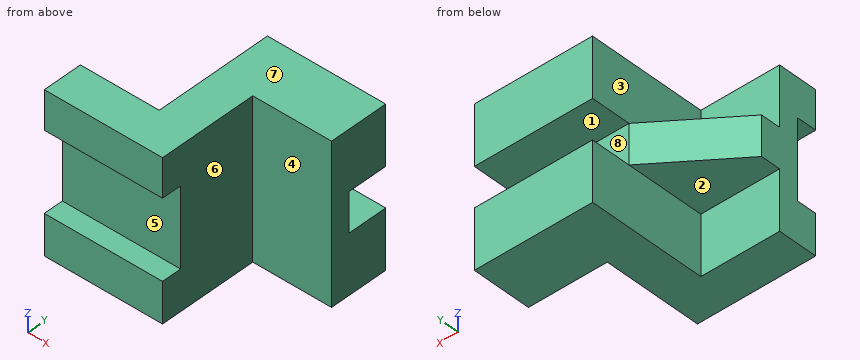
from build123d import *

# Parameters (mm, degrees)
BOSS_EXTRUDE1_DEPTH = 40
CUT_EXTRUDE1_DEPTH  = 30
CUT_EXTRUDE2_DEPTH  = 30
CUT_EXTRUDE3_REACH  = 62
SKETCH4_W           = 20
SKETCH4_H           = 20.212765958
CUT_EXTRUDE4_REACH  = 102
SKETCH5_W           = 40
SKETCH5_H           = 10


with BuildPart() as part:
    # Sketch1 → Boss-Extrude1 (new body, symmetric)
    with BuildSketch(Plane.XY):
        Polygon((-14.731740416, -28.723404255), (-14.731740416, 11.063829787), (-14.731740416, 31.276595745), (45.268259584, 31.276595745), (45.268259584, 1.276595745), (5.268259584, 1.276595745), (5.268259584, -48.723404255), (-54.731740416, -48.723404255), (-54.731740416, -28.723404255), align=None)
        Polygon((-54.731740416, -28.723404255), (-14.731740416, -28.723404255), (-14.731740416, 11.063829787), (-54.731740416, -18.723404255), align=None)
    extrude(amount=BOSS_EXTRUDE1_DEPTH, both=True)

    # Sketch2 → Cut-Extrude1 (cut)
    with BuildSketch(Plane.XY.offset(40)):
        Polygon((-54.731740416, -18.723404255), (-54.731740416, -28.723404255), (-14.731740416, -28.723404255), (-14.731740416, 11.063829787), align=None)
    extrude(amount=-CUT_EXTRUDE1_DEPTH, mode=Mode.SUBTRACT)

    # Sketch3 → Cut-Extrude2 (cut)
    with BuildSketch(Plane(origin=(0, 0, -40), x_dir=(-1, 0, 0), z_dir=(0, 0, -1))):
        Polygon((14.731740416, 11.063829787), (54.731740416, -18.723404255), (54.731740416, -28.723404255), (14.731740416, -28.723404255), align=None)
    extrude(amount=-CUT_EXTRUDE2_DEPTH, mode=Mode.SUBTRACT)

    # Sketch4 → Cut-Extrude3 (cut, up to next)
    with BuildSketch(Plane.ZY.offset(14.731740416), mode=Mode.PRIVATE) as cut_extrude3_sk1:
        with Locations((0, 21.170212766)):
            Rectangle(SKETCH4_W, SKETCH4_H)
    cut_extrude3_tool1 = extrude(cut_extrude3_sk1.sketch, amount=-CUT_EXTRUDE3_REACH, mode=Mode.PRIVATE) & part.part
    add(cut_extrude3_tool1.solids().sort_by_distance((-14.73174, 21.170213, 0))[0], mode=Mode.SUBTRACT)

    # Sketch5 → Cut-Extrude4 (cut, up to next)
    with BuildSketch(Plane.ZY.offset(54.731740416), mode=Mode.PRIVATE) as cut_extrude4_sk1:
        with Locations((0.497624841, -43.723404255)):
            Rectangle(SKETCH5_W, SKETCH5_H)
    cut_extrude4_tool1 = extrude(cut_extrude4_sk1.sketch, amount=-CUT_EXTRUDE4_REACH, mode=Mode.PRIVATE) & part.part
    add(cut_extrude4_tool1.solids().sort_by_distance((-54.73174, -43.723404, 0.497625))[0], mode=Mode.SUBTRACT)


solid = part.part
Geometry: final body of the model. Coordinates: model frame, mm. Face numbers are marked on the shaded views. A direction names the side the tool comes from. Coordinates: 2 decimals unless noted, no trailing zeros. Order: outer loops, then holes, each group sorted by start corner. A loop starts at its lowest first (then second) coordinate and runs counter-clockwise, first axis right, second up.
1) First-contact query: P1, Ø20, axis at x = 34, z = -17.5, coming from the -Y side; P2, Ø3, axis at y = -7, z = -11, coming from the +X side; P3, Ø12, axis at x = 10.5, z = 31.5, coming from the -Y side; P4, Ø20, axis at x = -26.5, y = -10.5, coming from the +Z side. Flat tips, straight axial feed; report the tip coordinate or a pass-through.
Result sheet:
P1: stops at y = 1.28
P2: stops at x = 5.27
P3: stops at y = -48.72
P4: stops at z = 10
2) Section A-A (y = 22.5). Return loops of the section in (x, z), then the cut area to 3 significant figures.
Result sheet:
outline: (-14.73, -40) - (45.27, -40) - (45.27, -10) - (-14.73, -10) - close; (-14.73, 10) - (45.27, 10) - (45.27, 40) - (-14.73, 40) - close
area: 3,600 mm2
3) Set-up query: the marked faces 1, 2, 3 and 4. Return all of +Z, -Z, +X, -X, +Y, -Y with unobstructed straight access to the full face (end or side cutting, diameter ignored); none if empty.
Result sheet:
face 1: +X, -X, +Y
face 2: -Z, -X, +Y
face 3: +Z, -X, +Y
face 4: +Z, -Z, +X, -Y
4) Section C-C (y = -22.5). Return loops of the section in (x, z), then the cut area to 3 significant figures.
Result sheet:
outline: (-54.73, -10) - (-14.73, -10) - (-14.73, -40) - (5.27, -40) - (5.27, 40) - (-14.73, 40) - (-14.73, 10) - (-54.73, 10) - close
area: 2,400 mm2
5) Draft query along Z for the marked faces 5, 6, 7 and 8. Return one class per face: released by +Z, released by -Z, zero draft, split by the parting line, or undercut.
Result sheet:
face 5: undercut
face 6: zero draft
face 7: released by +Z
face 8: undercut
6) Ray query, probe 1 along Z at (x, y) = (34, 17); probe 2 along Z at (x, y) = (-37, -45); probe 3 along Y at (x, z) = (-50, 30.5). Return the intervals inside material, ascending.
Result sheet:
probe 1: z = -40 to -10, 10 to 40
probe 2: z = -40 to -19.5, 20.5 to 40
probe 3: y = -48.72 to -28.72
7) Section B-B (z = -5.5). Return loops of the section in (x, y), then the cut area to 3 significant figures.
Result sheet:
outline: (-54.73, -38.72) - (5.27, -38.72) - (5.27, 1.28) - (45.27, 1.28) - (45.27, 11.06) - (-14.73, 11.06) - (-54.73, -18.72) - close
area: 2,780 mm2
8) Section D-D (x = -46.5). Return loops of the section in (y, z).
Result sheet:
outline: (-48.72, -40) - (-28.72, -40) - (-28.72, -10) - (-12.59, -10) - (-12.59, 10) - (-28.72, 10) - (-28.72, 40) - (-48.72, 40) - (-48.72, 20.5) - (-38.72, 20.5) - (-38.72, -19.5) - (-48.72, -19.5) - close
